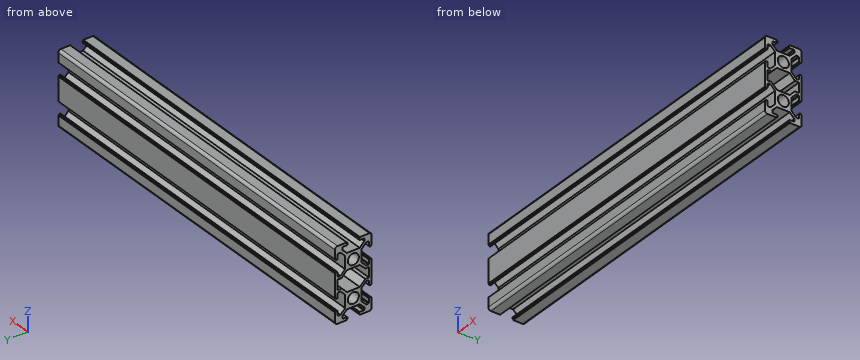
```python
from build123d import *

# Parameters (mm, degrees)
SKETCH_1_R      = 3
EXTRUDE_1_DEPTH = 200


with BuildPart() as part:
    # Эскиз1 → Бобышка-Вытянуть1 (new body)
    with BuildSketch(Plane(origin=(0, 0, 0), x_dir=(0, 0, -1), z_dir=(1, 0, 0))):
        with BuildLine():
            Line((19.519439061, 34.299030696), (24.519439061, 34.299030696))
            Line((24.519439061, 34.299030696), (27.319439061, 34.299030696))
            Line((27.319439061, 34.299030696), (32.319439061, 34.299030696))
            Line((32.319439061, 34.299030696), (32.319439061, 33.799030696))
            Line((32.319439061, 33.799030696), (32.819439061, 33.799030696))
            Line((32.819439061, 33.799030696), (32.819439061, 33.123453071))
            Line((32.819439061, 33.123453071), (32.470086687, 32.799030696))
            Line((32.470086687, 32.799030696), (30.231003523, 32.799030696))
            Line((30.231003523, 32.799030696), (29.919439061, 32.509699663))
            Line((29.919439061, 32.509699663), (29.919439061, 31.288014106))
            Line((29.919439061, 31.288014106), (32.444289636, 28.799030696))
            Line((32.444289636, 28.799030696), (39.394588486, 28.799030696))
            Line((39.394588486, 28.799030696), (41.919439061, 31.288014106))
            Line((41.919439061, 31.288014106), (41.919439061, 32.509699663))
            Line((41.919439061, 32.509699663), (41.607874598, 32.799030696))
            Line((41.607874598, 32.799030696), (39.368791434, 32.799030696))
            Line((39.368791434, 32.799030696), (39.019439061, 33.123453071))
            Line((39.019439061, 33.123453071), (39.019439061, 33.799030696))
            Line((39.019439061, 33.799030696), (39.519439061, 33.799030696))
            Line((39.519439061, 33.799030696), (39.519439061, 34.299030696))
            Line((39.519439061, 34.299030696), (44.519439061, 34.299030696))
            ThreePointArc((44.519439061, 34.299030696), (45.509388554, 33.88898019), (45.919439061, 32.899030696))
            Line((45.919439061, 32.899030696), (45.919439061, 27.899030696))
            Line((45.919439061, 27.899030696), (45.419439061, 27.899030696))
            Line((45.419439061, 27.899030696), (45.419439061, 27.399030696))
            Line((45.419439061, 27.399030696), (44.743861436, 27.399030696))
            Line((44.743861436, 27.399030696), (44.419439061, 27.748383069))
            Line((44.419439061, 27.748383069), (44.419439061, 29.987466234))
            Line((44.419439061, 29.987466234), (44.130108028, 30.299030696))
            Line((44.130108028, 30.299030696), (42.908422471, 30.299030696))
            Line((42.908422471, 30.299030696), (40.419439061, 27.774180121))
            Line((40.419439061, 27.774180121), (40.419439061, 20.823881271))
            Line((40.419439061, 20.823881271), (42.908422471, 18.299030696))
            Line((42.908422471, 18.299030696), (44.130108028, 18.299030696))
            Line((44.130108028, 18.299030696), (44.419439061, 18.610595158))
            Line((44.419439061, 18.610595158), (44.419439061, 20.849678323))
            Line((44.419439061, 20.849678323), (44.743861436, 21.199030696))
            Line((44.743861436, 21.199030696), (45.419439061, 21.199030696))
            Line((45.419439061, 21.199030696), (45.419439061, 20.699030696))
            Line((45.419439061, 20.699030696), (45.919439061, 20.699030696))
            Line((45.919439061, 20.699030696), (45.919439061, 15.699030696))
            ThreePointArc((45.919439061, 15.699030696), (45.509388554, 14.709081202), (44.519439061, 14.299030696))
            Line((44.519439061, 14.299030696), (39.519439061, 14.299030696))
            Line((39.519439061, 14.299030696), (39.519439061, 14.799030696))
            Line((39.519439061, 14.799030696), (39.019439061, 14.799030696))
            Line((39.019439061, 14.799030696), (39.019439061, 15.47460832))
            Line((39.019439061, 15.47460832), (39.368791434, 15.799030696))
            Line((39.368791434, 15.799030696), (41.607874598, 15.799030696))
            Line((41.607874598, 15.799030696), (41.919439061, 16.088361729))
            Line((41.919439061, 16.088361729), (41.919439061, 17.310047285))
            Line((41.919439061, 17.310047285), (39.394588486, 19.799030696))
            Line((39.394588486, 19.799030696), (32.444289636, 19.799030696))
            Line((32.444289636, 19.799030696), (29.919439061, 17.310047285))
            Line((29.919439061, 17.310047285), (29.919439061, 16.088361729))
            Line((29.919439061, 16.088361729), (30.231003523, 15.799030696))
            Line((30.231003523, 15.799030696), (32.470086687, 15.799030696))
            Line((32.470086687, 15.799030696), (32.819439061, 15.47460832))
            Line((32.819439061, 15.47460832), (32.819439061, 14.799030696))
            Line((32.819439061, 14.799030696), (32.319439061, 14.799030696))
            Line((32.319439061, 14.799030696), (32.319439061, 14.299030696))
            Line((32.319439061, 14.299030696), (27.319439061, 14.299030696))
            Line((27.319439061, 14.299030696), (24.519439061, 14.299030696))
            Line((24.519439061, 14.299030696), (19.519439061, 14.299030696))
            Line((19.519439061, 14.299030696), (19.519439061, 14.799030696))
            Line((19.519439061, 14.799030696), (19.019439061, 14.799030696))
            Line((19.019439061, 14.799030696), (19.019439061, 15.47460832))
            Line((19.019439061, 15.47460832), (19.368791434, 15.799030696))
            Line((19.368791434, 15.799030696), (21.607874598, 15.799030696))
            Line((21.607874598, 15.799030696), (21.919439061, 16.088361729))
            Line((21.919439061, 16.088361729), (21.919439061, 17.310047285))
            Line((21.919439061, 17.310047285), (19.394588486, 19.799030696))
            Line((19.394588486, 19.799030696), (12.444289636, 19.799030696))
            Line((12.444289636, 19.799030696), (9.919439061, 17.310047285))
            Line((9.919439061, 17.310047285), (9.919439061, 16.088361729))
            Line((9.919439061, 16.088361729), (10.231003523, 15.799030696))
            Line((10.231003523, 15.799030696), (12.470086687, 15.799030696))
            Line((12.470086687, 15.799030696), (12.819439061, 15.47460832))
            Line((12.819439061, 15.47460832), (12.819439061, 14.799030696))
            Line((12.819439061, 14.799030696), (12.319439061, 14.799030696))
            Line((12.319439061, 14.799030696), (12.319439061, 14.299030696))
            Line((12.319439061, 14.299030696), (7.319439061, 14.299030696))
            ThreePointArc((7.319439061, 14.299030696), (6.329489567, 14.709081202), (5.919439061, 15.699030696))
            Line((5.919439061, 15.699030696), (5.919439061, 20.699030696))
            Line((5.919439061, 20.699030696), (6.419439061, 20.699030696))
            Line((6.419439061, 20.699030696), (6.419439061, 21.199030696))
            Line((6.419439061, 21.199030696), (7.095016685, 21.199030696))
            Line((7.095016685, 21.199030696), (7.419439061, 20.849678323))
            Line((7.419439061, 20.849678323), (7.419439061, 18.610595158))
            Line((7.419439061, 18.610595158), (7.708770093, 18.299030696))
            Line((7.708770093, 18.299030696), (8.93045565, 18.299030696))
            Line((8.93045565, 18.299030696), (11.419439061, 20.823881271))
            Line((11.419439061, 20.823881271), (11.419439061, 27.774180121))
            Line((11.419439061, 27.774180121), (8.93045565, 30.299030696))
            Line((8.93045565, 30.299030696), (7.708770093, 30.299030696))
            Line((7.708770093, 30.299030696), (7.419439061, 29.987466234))
            Line((7.419439061, 29.987466234), (7.419439061, 27.748383069))
            Line((7.419439061, 27.748383069), (7.095016685, 27.399030696))
            Line((7.095016685, 27.399030696), (6.419439061, 27.399030696))
            Line((6.419439061, 27.399030696), (6.419439061, 27.899030696))
            Line((6.419439061, 27.899030696), (5.919439061, 27.899030696))
            Line((5.919439061, 27.899030696), (5.919439061, 32.899030696))
            ThreePointArc((5.919439061, 32.899030696), (6.329489567, 33.88898019), (7.319439061, 34.299030696))
            Line((7.319439061, 34.299030696), (12.319439061, 34.299030696))
            Line((12.319439061, 34.299030696), (12.319439061, 33.799030696))
            Line((12.319439061, 33.799030696), (12.819439061, 33.799030696))
            Line((12.819439061, 33.799030696), (12.819439061, 33.123453071))
            Line((12.819439061, 33.123453071), (12.470086687, 32.799030696))
            Line((12.470086687, 32.799030696), (10.231003523, 32.799030696))
            Line((10.231003523, 32.799030696), (9.919439061, 32.509699663))
            Line((9.919439061, 32.509699663), (9.919439061, 31.288014106))
            Line((9.919439061, 31.288014106), (12.444289636, 28.799030696))
            Line((12.444289636, 28.799030696), (19.394588486, 28.799030696))
            Line((19.394588486, 28.799030696), (21.919439061, 31.288014106))
            Line((21.919439061, 31.288014106), (21.919439061, 32.509699663))
            Line((21.919439061, 32.509699663), (21.607874598, 32.799030696))
            Line((21.607874598, 32.799030696), (19.368791434, 32.799030696))
            Line((19.368791434, 32.799030696), (19.019439061, 33.123453071))
            Line((19.019439061, 33.123453071), (19.019439061, 33.799030696))
            Line((19.019439061, 33.799030696), (19.519439061, 33.799030696))
            Line((19.519439061, 33.799030696), (19.519439061, 34.299030696))
        make_face()
        with Locations((15.919439061, 24.299030696)):
            Circle(SKETCH_1_R, mode=Mode.SUBTRACT)
        with Locations((35.919439061, 24.299030696)):
            Circle(SKETCH_1_R, mode=Mode.SUBTRACT)
        Polygon((28.627102151, 32.799030696), (23.21177597, 32.799030696), (23.21177597, 30.602545824), (20.272319384, 27.774180121), (20.272319384, 20.823881271), (23.21177597, 17.768970439), (23.21177597, 15.799030696), (28.627102151, 15.799030696), (28.627102151, 17.768970439), (31.566558738, 20.823881271), (31.566558738, 27.774180121), (28.627102151, 30.602545824), align=None, mode=Mode.SUBTRACT)
    extrude(amount=EXTRUDE_1_DEPTH)


solid = part.part
```
Input: part model. Units: mm. Frame: model coordinates. Coordinates: 2 decimals unless noted, no trailing zeros. Answer as a JSON object with one key per item and string values.
1. First-contact query: P1, Ø1.5, axis at y = 25.5, z = -37, coming from the -X side; P2, Ø0.5, axis at x = 107, y = 15, coming from the +Z side; P3, Ø2, axis at x = 66, z = -35.5, coming from the -Y side; P4, Ø0.6, axis at x = 68, y = 34, coming from the +Z side. Flat tips, straight axial feed; report the tip coordinate or a pass-through.
Result set:
{"P1": "passes through", "P2": "stops at z = -5.99", "P3": "stops at y = 19.8", "P4": "stops at z = -6.17"}
2. Section A-A on x = 158. Count the separate pieces of the cut face and the enclosed holes in it, then the cut area to 3 significant figures.
Result set:
{"separate pieces": "1", "enclosed holes": "3", "area": "282 mm2"}
3. Material intervals for line 1 (Y direction, x = 96, z = -12.5); line 2 (Z direction, x = 97.5, y = 21); line 3 (Z direction, x = 44.5, y = 19.5), sorted ascending. Write a range as from..to.
Result set:
{"line 1": "y = 14.8..15.77, 19.8..28.8, 32.83..33.8", "line 2": "z = -45.42..-44.56, -40.42..-31.57, -20.27..-11.42, -7.28..-6.42", "line 3": "z = -45.92..-44.42, -41.72..-39.7, -32.14..-30.29, -21.55..-19.7, -12.14..-10.11, -7.42..-5.92"}
